The listing builds one solid part. Answer for the finished solid, in the listing's coordinates (mm). Give positions to 0.01 mm unless a question says otherwise; leave off trailing zeros. Order: outer loops, then holes, each group sorted by start corner. A loop starts at its lowest first (then second) coordinate and runs counter-clockwise, first axis right, second up. Notation, with made-up numbers: (-32.5, 78.5) - (13.5, 78.5) arc R29 ccw to (13.5, 108.5) - close; hole circle Ø6 at (67.25, 31). An arc over 180 degrees is marked (long way). Answer as a JSON object with one key per item and string values. Group by question number.
Q1. A cutting plane is placed at C-C, the plane y = 5.3. Give the vertices of the cut face in (x, z), and give its area (3 significant figures).
Q2. Given pin 1 (2 mm diameter, centred on x = 6.5, y = 4, fed in from -Z), flat-ended and moving along its own axis, determine where the tip first touches the part or whether it passes through.
Q3. A cutting plane is placed at A-A, the plane x = 5.8. Give the vertices of the cut face in (y, z).
Q4. A cutting plane is placed at D-D, the plane x = 10.5. Give the vertices of the cut face in (y, z), and give its area (3 significant figures).
Q5. A cutting plane is placed at B-B, the plane z = 0.3. Give the vertices of the cut face in (x, y), and give its area (3 significant figures).
Q6. The mould has two halves that part along Y. Classify faces 1 (the face through (6, 4, 1)), 2 (the face through (0.767, 9.873, 0.507)), 3 (the face through (5.8, 5.8, 0.5)): released by +Y, released by -Y, zero draft, split by the parting line, or undercut.
Q7. Consider line 1 (X direction, y = 5.3, z = 0.4); line 2 (Y direction, x = 5.8, z = 0.65); line 3 (Y direction, x = 10.25, z = 0.5). Determine where each line is inside the solid, lowest interval first.
Autodesk Inventor part; units mm, degrees
ref_plane "YZ Plane" through (0, 0, 0) normal (1, 0, 0) x (0, 1, 0)
ref_plane "XZ Plane" through (0, 0, 0) normal (0, 1, 0) x (-1, 0, 0)
ref_plane "XY Plane" through (0, 0, 0) normal (0, 0, 1) x (1, 0, 0)
sketch "Эскиз1" plane through (0, 0, 0) normal (0, 0, 1) x (1, 0, 0)
  line L0 (0, 0) -> (11.6, 0)
  line L1 (11.6, 0) -> (11.6, 10.6)
  line L2 (11.6, 10.6) -> (0, 10.6)
  line L3 (0, 10.6) -> (0, 0)
  dimension "d0" = 11.6
  dimension "d1" = 10.6
extrude "Выдавливание1" add sketch "Эскиз1" along normal blind 1
fillet "Сопряжение1" radius 2.55 2 edges at (11.6, 10.6, 0.5) (0, 10.6, 0.5)
sketch "Эскиз2" plane through (0, 0, 1) normal (0, 0, 1) x (1, 0, 0)
  line L0 (0, 0) -> (11.6, 0)
  line L1 (5.8, 0) -> (5.8, 10.6)
  line L2 (9.05, 10.6) -> (2.55, 10.6)
  point P0 (5.8, 5.3)
hole "Отверстие1" at (5.8, 5.3, 1) direction (0, 0, -1) diameter 1 end through all
properties part number "Encoder"
Reply:
{
 "1": {"outline": "(0, 0) - (5.3, 0) - (5.3, 1) - (0, 1) - close; (6.3, 0) - (11.6, 0) - (11.6, 1) - (6.3, 1) - close", "area": "10.6 mm^2"},
 "2": {"pin 1": "stops at z = 0"},
 "3": {"outline": "(0, 0) - (4.8, 0) - (4.8, 1) - (0, 1) - close; (5.8, 0) - (10.6, 0) - (10.6, 1) - (5.8, 1) - close"},
 "4": {"outline": "(0, 0) - (10.15, 0) - (10.15, 1) - (0, 1) - close", "area": "10.1 mm^2"},
 "5": {"outline": "(0, 0) - (11.6, 0) - (11.6, 8.05) arc R2.55 ccw to (9.05, 10.6) - (2.55, 10.6) arc R2.55 ccw to (0, 8.05) - close; hole circle Ø1 at (5.8, 5.3)", "area": "119 mm^2"},
 "6": {"face 1": "zero draft", "face 2": "released by +Y", "face 3": "undercut"},
 "7": {"line 1": "x = 0 to 5.3, 6.3 to 11.6", "line 2": "y = 0 to 4.8, 5.8 to 10.6", "line 3": "y = 0 to 10.3"}
}
